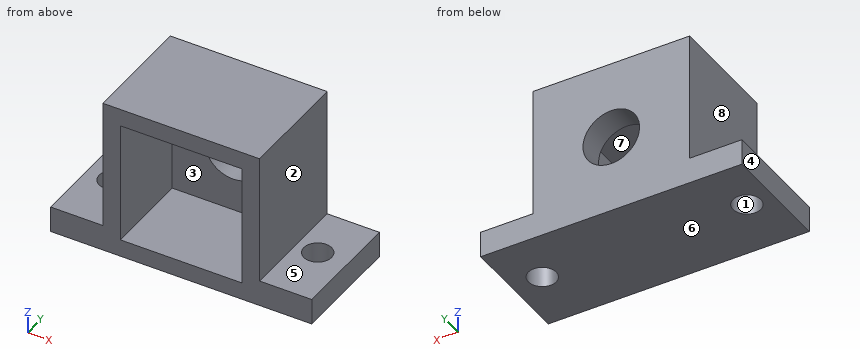
```python
from build123d import *

# Parameters (mm, degrees)
SKETCH_R     = 3.25
PAD_DEPTH    = 3
SKETCH001_W  = 14
SKETCH001_H  = 14
PAD001_DEPTH = 13
SKETCH002_R  = 1.6
POCKET_DEPTH = 18.001


with BuildPart() as part:
    # Sketch → Pad (new body)
    with BuildSketch(Plane.XZ):
        Polygon((0, 0), (30, 0), (30, 3), (24, 3), (24, 18), (6, 18), (6, 3), (0, 3), align=None)
        with Locations((15, 9)):
            Circle(SKETCH_R, mode=Mode.SUBTRACT)
    extrude(amount=PAD_DEPTH)

    # Sketch001 → Pad001 (join)
    with BuildSketch(Plane.XZ):
        Polygon((0, 0), (0, 3), (6, 3), (6, 18), (24, 18), (24, 3), (30, 3), (30, 0), align=None)
        with Locations((15, 9)):
            Rectangle(SKETCH001_W, SKETCH001_H, mode=Mode.SUBTRACT)
    extrude(amount=PAD001_DEPTH)

    # Sketch002 → Pocket (cut, through all)
    with BuildSketch(Plane.XY):
        with Locations((3, -6)):
            Circle(SKETCH002_R)
        with Locations((26.5, -6)):
            Circle(SKETCH002_R)
    extrude(amount=POCKET_DEPTH, mode=Mode.SUBTRACT)


solid = part.part
```
Input: part model. Units: mm. Frame: model coordinates. Face numbers are marked on the shaded views. A direction names the side the tool comes from. Round coordinates to 2 decimals unless told otherwise and drop trailing zeros. Loops run counter-clockwise (first coordinate to the right, second up) from the corner with the lowest first, then second, coordinate; pieces in that order, holes last.
1) Section query D-D on y = -8.25. Return the cut outline in (x, z).
Ans:
outline: (0, 0) - (30, 0) - (30, 3) - (24, 3) - (24, 18) - (6, 18) - (6, 3) - (0, 3) - close; hole (8, 2) - (22, 2) - (22, 16) - (8, 16) - close
2) Pin query (flat end, axial travel): pin 1 (1.9 mm diameter, centred on x = 3, y = -6, fed in from +Z); pin 2 (6 mm diameter, centred on y = -7, z = 12.5, fed in from +X); pin 3 (1.5 mm diameter, centred on y = -2.5, z = 15, fed in from -X); pin 4 (10.5 mm diameter, centred on x = 15, z = 9, fed in from -Y). Return the tip coordinate at first contact, or that it passes through.
Ans:
pin 1: passes through
pin 2: stops at x = 24
pin 3: stops at x = 6
pin 4: stops at y = -3
3) Material intervals for line 1 (Z direction, x = 16.75, y = -5.5); line 2 (X direction, y = -10.25, z = 5.25); line 3 (Y direction, x = 26.5, z = 2.3), sorted ascending.
Ans:
line 1: z = 0 to 2, 16 to 18
line 2: x = 6 to 8, 22 to 24
line 3: y = -13 to -7.6, -4.4 to 0
4) Section query C-C on z = 9. Return the cut outline in (x, y).
Ans:
outline: (6, -13) - (8, -13) - (8, -3) - (11.75, -3) - (11.75, 0) - (6, 0) - close; (18.25, -3) - (22, -3) - (22, -13) - (24, -13) - (24, 0) - (18.25, 0) - close
5) Section query B-B on x = 3. Return the cut outline in (y, z), plus the area to 3 significant figures.
Ans:
outline: (-13, 0) - (-7.6, 0) - (-7.6, 3) - (-13, 3) - close; (-4.4, 0) - (0, 0) - (0, 3) - (-4.4, 3) - close
area: 29.4 mm2
6) Pull-direction query (X, two-part tool) for the marked faces 1, 2, 3 and 4; classes: released by +X, released by -X, zero draft, split by the parting line, or undercut.
Ans:
face 1: undercut
face 2: released by +X
face 3: undercut
face 4: released by -X
7) Section query A-A on y = -6. Return the cut outline in (x, z).
Ans:
outline: (0, 0) - (1.4, 0) - (1.4, 3) - (0, 3) - close; (4.6, 0) - (24.9, 0) - (24.9, 3) - (24, 3) - (24, 18) - (6, 18) - (6, 3) - (4.6, 3) - close; (28.1, 0) - (30, 0) - (30, 3) - (28.1, 3) - close; hole (8, 2) - (22, 2) - (22, 16) - (8, 16) - close
8) Set-up query: the marked faces 5, 6, 7 and 8. Return all of +Z, -Z, +X, -X, +Y, -Y with unobstructed straight access to the full face (end or side cutting, diameter ignored); none if empty.
Ans:
face 5: +Z, +X, +Y, -Y
face 6: -Z, +X, -X, +Y, -Y
face 7: -Y
face 8: +Z, -X, +Y, -Y
